from build123d import *

# Parameters (mm, degrees)
F1_DEPTH = 203.2
F3_DEPTH = 3.302


with BuildPart() as f1:
    # F0 (on Right) → F1 (new body, symmetric)
    with BuildSketch(Plane.YZ):
        Polygon((38.1, 0), (-38.1, 0), (-38.1, -38.1), (-33.02, -38.1), (-33.02, -3.302), (33.02, -3.302), (33.02, -38.1), (38.1, -38.1), align=None)
    extrude(amount=F1_DEPTH, both=True)

    # F2 (on face) → F3 (cut, through all)
    with BuildSketch(Plane.XY):
        with BuildLine():
            Line((187.325, 17.78), (193.675, 17.78))
            ThreePointArc((193.675, 17.78), (195.920064, 18.709936), (196.85, 20.955))
            ThreePointArc((196.85, 20.955), (195.920064, 23.200064), (193.675, 24.13))
            Line((193.675, 24.13), (187.325, 24.13))
            ThreePointArc((187.325, 24.13), (185.079936, 23.200064), (184.15, 20.955))
            ThreePointArc((184.15, 20.955), (185.079936, 18.709936), (187.325, 17.78))
        make_face()
        with BuildLine():
            ThreePointArc((196.85, -20.955), (195.920064, -18.709936), (193.675, -17.78))
            Line((193.675, -17.78), (187.325, -17.78))
            ThreePointArc((187.325, -17.78), (185.079936, -18.709936), (184.15, -20.955))
            ThreePointArc((184.15, -20.955), (185.079936, -23.200064), (187.325, -24.13))
            Line((187.325, -24.13), (193.675, -24.13))
            ThreePointArc((193.675, -24.13), (195.920064, -23.200064), (196.85, -20.955))
        make_face()
    extrude(amount=-F3_DEPTH, mode=Mode.SUBTRACT)


solid = f1.part
Here's how the part is built. I have some questions about the finished solid (model axes, mm). A direction names the side the tool comes from. Coordinates: 2 decimals unless noted, no trailing zeros. Order: outer loops, then holes, each group sorted by start corner. A loop starts at its lowest first (then second) coordinate and runs counter-clockwise, first axis right, second up. Notation, with made-up numbers: M 41,-2 L 50,-2 A30 cw 50,23 Z; hole C 86.25,72.25 d5. An arc over 180 degrees is marked long. Answer as CSV lines item,"result". Start each with the question number.
1. I need wall thicknesses on line 1 (Y direction, x = -178, z = -30.5); line 2 (Z direction, x = 96.5, y = 14). Which ranges of each line are inside material? Lowest first, please. Write a range as [from, to].
2. On a 3-axis mill with a long thin cutter (end or side, diameter ignored), from which of +Z, -Z, +X, -X, +Y, -Y can I reach the whole of each face in a straight line? I mean faces 4 (the flat face through (3, 0, -3.302)), 5 (the flat face through (203.2, -6, -2)). Say none if no direction works.
3. I want a section at B-B, the plane x = 170. Write out the boundary of the cut face in (y, z), and give its area (3 significant figures).
4. For pin 1 (5 mm diameter, centred on y = 7.5, z = -4.5, fed in from +X), with a flat end and sliding along its axis, tell me the tip position at first contact or that it passes through.
5. We'd pull the mould along Y, two halves only. Please class faces 1 (the flat face through (3, -33.02, -21)), 2 (the flat face through (3, 1, 0)), 3 (the flat face through (3, -38.1, -19)): released by +Y, released by -Y, zero draft, split by the parting line, or undercut.
6. I want a section at A-A, the plane z = -33. Write out the boundary of the cut face in (x, y), and give its area (3 significant figures).
7. I want a section at C-C, the plane y = -8. Write out the boundary of the cut face in (x, z).
Recorded:
1,line 1,"y = [-38.1, -33.02], [33.02, 38.1]"
1,line 2,"z = [-3.3, 0]"
2,face 4,"-Z, +X, -X"
2,face 5,"+Z, -Z, +X, +Y, -Y"
3,outline,"M -38.1,-38.1 L -33.02,-38.1 L -33.02,-3.3 L 33.02,-3.3 L 33.02,-38.1 L 38.1,-38.1 L 38.1,0 L -38.1,0 Z"
3,area,"605 mm2"
4,pin 1,"stops at x = 203.2"
5,face 1,"undercut"
5,face 2,"zero draft"
5,face 3,"released by -Y"
6,outline,"M -203.2,-38.1 L 203.2,-38.1 L 203.2,-33.02 L -203.2,-33.02 Z; M -203.2,33.02 L 203.2,33.02 L 203.2,38.1 L -203.2,38.1 Z"
6,area,"4,130 mm2"
7,outline,"M -203.2,-3.3 L 203.2,-3.3 L 203.2,0 L -203.2,0 Z"
